Autodesk Inventor part; units mm, degrees
ref_plane "YZ Plane" through (0, 0, 0) normal (1, 0, 0) x (0, 1, 0)
ref_plane "XZ Plane" through (0, 0, 0) normal (0, 1, 0) x (-1, 0, 0)
ref_plane "XY Plane" through (0, 0, 0) normal (0, 0, 1) x (1, 0, 0)
sketch "Sketch1" plane through (0, 0, 0) normal (0, 1, 0) x (-1, 0, 0)
  line L0 (0, 0) -> (0, -20)
  line L1 (0, 0) -> (-4, 0) construction
  line L2 (0, -20) -> (-4, -20) construction
  line L3 (0, 0) -> (-5, 0)
  arc A0 (5, 0) -> (-5, 0) centre (0, 0) ccw
  line L4 (-5, 0) -> (-5, -20)
  arc A1 (-5, -20) -> (5, -20) centre (0, -20) ccw
  line L5 (5, -20) -> (5, 0)
  dimension "d11" = 20
  dimension "d12" = 5
  dimension "d13" = 90
  dimension "d14" = 20
sketch "Sketch1 outline for Extrusion1" plane through (0, 0, 0) normal (0, 1, 0) x (-1, 0, 0)
  arc A0 (-5, 0) -> (5, 0) centre (0, 0) cw
  line L0 (5, 0) -> (5, -20)
  arc A1 (5, -20) -> (-5, -20) centre (0, -20) cw
  line L1 (-5, -20) -> (-5, 0)
extrude "Extrusion1" add sketch "Sketch1 outline for Extrusion1" along normal blind 5.5
sketch "Sketch2" plane through (0, 5.5, 0) normal (0, 1, 0) x (1, 0, 0)
  circle A0 centre (0, 0) radius 2.655
  line L0 (0, 0) -> (0, 20)
  circle A1 centre (0, 20) radius 2.655
  dimension "d7" = 5.31
  dimension "d8" = 20
  dimension "d9" = 5.31
sketch "Sketch3" plane through (0, 0, 0) normal (0, -1, 0) x (1, 0, 0)
  circle A0 centre (0, 0) radius 1.9
  line L0 (0, 0) -> (0, -20)
  circle A1 centre (0, -20) radius 1.9
  dimension "d15" = 3.8
  dimension "d16" = 20
  dimension "d17" = 3.8
sketch "Sketch3 outline for Extrusion2" plane through (0, 0, 0) normal (0, -1, 0) x (1, 0, 0)
  circle A0 centre (0, 0) radius 1.9
  circle A1 centre (0, -20) radius 1.9
extrude "Extrusion2" cut sketch "Sketch3 outline for Extrusion2" against normal blind 1.2
sketch "Sketch4" plane through (0, 1.2, -20) normal (0, -1, 0) x (1, 0, 0)
  circle A0 centre (0, 0) radius 1.9
  circle A1 centre (0, 0) radius 1.9
  circle A2 centre (0, 20) radius 1.9
sketch "Sketch5" plane through (5, 0, 0) normal (1, 0, 0) x (0, 0, -1)
  line L0 (0, 0) -> (0, 5.5)
  line L1 (0, 0) -> (0, 5.5)
hole "Hole1" at (0, 5.5, 0) at (0, 5.5, -20) direction (0, -1, 0) diameter 5.1 depth 4 tip angle 118 countersink diameter 5.31 countersink angle 3.01
thicken "Thicken1" operation add thickness 2 both sides no extend neighbours yes toward (0.9967573, 0, -0.0804666) faces at (4.983787, 3.666667, -20.402333) (5, 1.833333, -13.333333) (-5, 1.833333, -6.666667) (-4.983787, 3.666667, 0.402333)
properties part number "Rod_constraint"
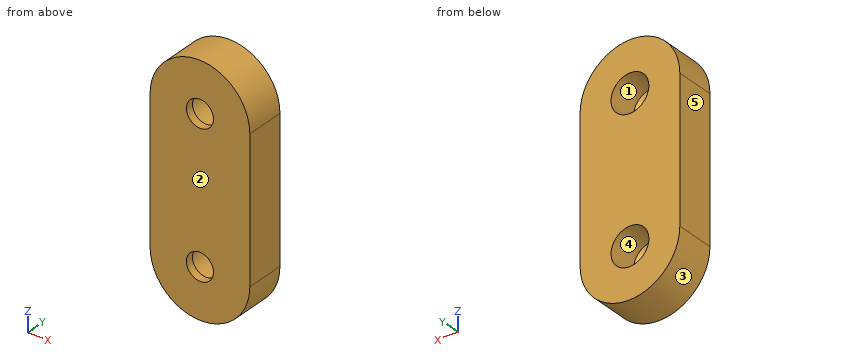
Work out the finished part from the listing and answer in its coordinate system (mm). Face numbers are marked on the shaded views. A direction names the side the tool comes from. Give positions to 0.01 mm unless a question says otherwise; leave off trailing zeros. Write each loop counter-clockwise with the first axis right and the second up, starting at its lowest first coordinate (ties: lowest second). Pieces come first, ordered by that corner, then holes. Notation, with made-up numbers: (87, 26.25) - (122, 26.25) arc R14 cw to (122, 52.25) - close; hole circle Ø10 at (-3, 38.25). An arc over 180 degrees is marked (long way). One line per item, written item: value. Start each with the question number.
1. Find section A-A (x = 0). State how many separate pieces and enclosed holes the cut face has, then the cut area to 3 significant figures.
2. Given pin 1 (3 mm diameter, centred on x = -3, y = 1, fed in from +Z); pin 2 (3.5 mm diameter, centred on x = 0, z = -20, fed in from -Y); pin 3 (1 mm diameter, centred on x = -5.5, y = 0.5, fed in from +Z); pin 4 (3 mm diameter, centred on x = 4.5, y = 4.5, fed in from -Z), each flat-ended and moving along its own axis, determine where each tip first touches the part or whether it passes through.
3. Find section C-C (z = 3.5). Write down the section's boundary in (x, y), then the cut area to 3 significant figures.
4. Find section B-B (y = 3.7). Write down the section's boundary in (x, z).
5. Consider probe 1 along Z at (x, y) = (0, 0.5); probe 2 along X at (y, z) = (1.55, -20); probe 3 along X at (y, z) = (0.6, 0). Determine where each line is inside the solid, lowest interval first.
6. For a pull along X with two mould halves and no side action, classify the marked faces 1, 2 and 3 as +X half, -X half, draft (parallel to the pull), parting line (faces both ways), or undercut.
7. For the marked faces 4 and 5, determine the directions among +Z, -Z, +X, -X, +Y, -Y from which every point of the face is accessible in a straight line to the end or side of a thin tool.
Geometry results:
1. separate pieces: 3
1. enclosed holes: 0
1. area: 133 mm2
2. pin 1: z = 6.84
2. pin 2: through
2. pin 3: z = 4.9
2. pin 4: z = -26.32
3. outline: (-6.06, 0) - (6.06, 0) - (6.06, 5.5) - (-6.06, 5.5) - close
3. area: 66.7 mm2
4. outline: (-7, -20) arc R7 ccw to (7, -20) - (7, 0) arc R7 ccw to (-7, 0) - close; hole circle Ø5.22 at (0, -20); hole circle Ø5.22 at (0, 0)
5. probe 1: -27 to -21.9, -18.1 to -1.9, 1.9 to 7
5. probe 2: -7 to -2.55, 2.55 to 7
5. probe 3: -7 to -1.9, 1.9 to 7
6. face 1: undercut
6. face 2: draft
6. face 3: parting line
7. face 4: +Y
7. face 5: +Z, -Z, -X, +Y, -Y
